Input: part model. Units: mm. Frame: model coordinates. A direction names the side the tool comes from. Give positions to 0.01 mm unless a question says otherwise; leave off trailing zeros. Loops run counter-clockwise (first coordinate to the right, second up) from the corner with the lowest first, then second, coordinate; pieces in that order, holes last. Notation, with made-up numbers: M 77.25,-38.5 L 112.25,-38.5 A18 cw 112.25,-11.5 Z; hole C -33,-28.5 d3. An arc over 180 degrees is marked long. Answer as a JSON object with one key per item and string values. Group by question number.
1) Access query for faces 1 (the flat face through (15, 27.633, 7)), 2 (the flat face through (0, 1, 0)). Directions: +Z, -Z, +X, -X, +Y, -Y. A direction counts if a zero-diameter tool reaches every point of the face in a straight line with its end or side. Return the directions, or none.
2) Draft query along X for faces 3 (the flat face through (15, 30, 6)), 4 (the flat face through (27, -1, 4)), 5 (the flat face through (0, 1, 8)). Return one class per face: +X half, -X half, draft (parallel to the pull), parting line (faces both ways), or undercut.
3) Section query C-C on x = 11.5. Return loops of the section in (y, z), plus the area to 3 significant figures.
4) Ray query, L1, parallel to X at y = 28, z = 7.5; L2, parallel to Z at x = 14, y = -22.5. Return the intervals inside material, ascending.
5) Section query B-B on y = 29. Return loops of the section in (x, z), plus the area to 3 significant figures.
6) Section query D-D on y = -21.5. Return loops of the section in (x, z).
7) Section query A-A on x = -20. Return loops of the section in (y, z).
8) First-contact query: P1, Ø0.5, axis at x = -18.5, z = 8.5, coming from the -Y side; P2, Ø5.5, axis at x = 16, y = -8, coming from the +Z side; P3, Ø1.1, axis at y = -8.5, z = 8.5, coming from the -X side; P4, Ø0.5, axis at y = 13.5, z = 8.5, coming from the +X side. Flat tips, straight axial feed; report the tip coordinate or a pass-through.
from build123d import *

# Parameters (mm, degrees)
F0_W     = 54
F0_H     = 80
F1_DEPTH = 8
F2_W     = 10
F2_H     = 5
F3_DEPTH = 1
F4_W     = 10
F4_H     = 5
F5_DEPTH = 2


with BuildPart() as f1:
    # F0 (on Top) → F1 (new body)
    with BuildSketch(Plane.XY):
        Rectangle(F0_W, F0_H)
    extrude(amount=F1_DEPTH)

    # F2 (on face) → F3 (join)
    with BuildSketch(Plane.XY.offset(8)):
        with Locations((-18.653328, 30.132598)):
            Rectangle(F2_W, F2_H)
        with Locations((-18.653328, 12.571623)):
            Rectangle(F2_W, F2_H)
        with Locations((-18.653328, -7.428377)):
            Rectangle(F2_W, F2_H)
    extrude(amount=F3_DEPTH)

    # F4 (on face) → F5 (cut)
    with BuildSketch(Plane.XY.offset(8)):
        with Locations((15.056205, 30.132598)):
            Rectangle(F4_W, F4_H)
        with Locations((15.056205, 12.571623)):
            Rectangle(F4_W, F4_H)
        with Locations((15.056205, -7.428377)):
            Rectangle(F4_W, F4_H)
    extrude(amount=-F5_DEPTH, mode=Mode.SUBTRACT)


solid = f1.part
Output:
{
 "1": {"face 1": "+Z", "face 2": "-Z, +X, -X, +Y, -Y"},
 "2": {"face 3": "undercut", "face 4": "+X half", "face 5": "draft"},
 "3": {"outline": "M -40,0 L 40,0 L 40,8 L 32.63,8 L 32.63,6 L 27.63,6 L 27.63,8 L 15.07,8 L 15.07,6 L 10.07,6 L 10.07,8 L -4.93,8 L -4.93,6 L -9.93,6 L -9.93,8 L -40,8 Z", "area": "610 mm^2"},
 "4": {"L1": "x = -27 to 10.06, 20.06 to 27", "L2": "z = 0 to 8"},
 "5": {"outline": "M -27,0 L 27,0 L 27,8 L 20.06,8 L 20.06,6 L 10.06,6 L 10.06,8 L -13.65,8 L -13.65,9 L -23.65,9 L -23.65,8 L -27,8 Z", "area": "422 mm^2"},
 "6": {"outline": "M -27,0 L 27,0 L 27,8 L -27,8 Z"},
 "7": {"outline": "M -40,0 L 40,0 L 40,8 L 32.63,8 L 32.63,9 L 27.63,9 L 27.63,8 L 15.07,8 L 15.07,9 L 10.07,9 L 10.07,8 L -4.93,8 L -4.93,9 L -9.93,9 L -9.93,8 L -40,8 Z"},
 "8": {"P1": "stops at y = -9.93", "P2": "stops at z = 8", "P3": "stops at x = -27", "P4": "stops at x = -13.65"}
}
